Work out the finished part from the listing and answer in its coordinate system (mm). Give positions to 0.01 mm unless a question says otherwise; leave off trailing zeros. Loops run counter-clockwise (first coordinate to the right, second up) from the corner with the lowest first, then second, coordinate; pieces in that order, holes last.
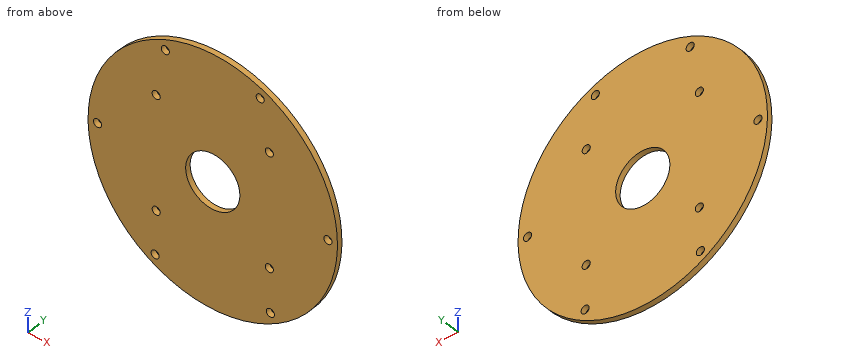
```python
from build123d import *

# Parameters (mm, degrees)
SKETCH_1_R          = 46
EXTRUDE_1_DEPTH     = 2
SKETCH_2_R          = 1.5
CUT_EXTRUDE_1_DEPTH = 66.084560381
SKETCH_3_R          = 1.5
CUT_EXTRUDE_2_DEPTH = 66.084560381
SKETCH_4_R          = 10
CUT_EXTRUDE_3_DEPTH = 66.084560381


with BuildPart() as part:
    # 草图1 → 凸台-拉伸1 (new body)
    with BuildSketch(Plane(origin=(0, 0, 0), x_dir=(1, 0, 0), z_dir=(0, 1, 0))):
        with Locations(Location((0, 0, 0), (0, 0, 270))):
            Circle(SKETCH_1_R)
    extrude(amount=EXTRUDE_1_DEPTH)

    # 草图2 → 切除-拉伸1 (cut, through all)
    with BuildSketch(Plane(origin=(0, 2, 0), x_dir=(1, 0, 0), z_dir=(0, 1, 0))):
        with Locations(Location((-21.25, 36.806079661, 0), (0, 0, 270))):
            Circle(SKETCH_2_R)
        with Locations(Location((21.25, 36.806079661, 0), (0, 0, 270))):
            Circle(SKETCH_2_R)
        with Locations(Location((42.5, 0, 0), (0, 0, 270))):
            Circle(SKETCH_2_R)
        with Locations(Location((-42.5, 0, 0), (0, 0, 270))):
            Circle(SKETCH_2_R)
        with Locations(Location((-17.5, -38.729833462, 0), (0, 0, 270))):
            Circle(SKETCH_2_R)
        with Locations(Location((17.5, -38.729833462, 0), (0, 0, 90))):
            Circle(SKETCH_2_R)
    extrude(amount=-CUT_EXTRUDE_1_DEPTH, mode=Mode.SUBTRACT)

    # 草图3 → 切除-拉伸2 (cut, through all)
    with BuildSketch(Plane(origin=(0, 2, 0), x_dir=(1, 0, 0), z_dir=(0, 1, 0))):
        with Locations(Location((-20.859650045, -20.859650045, 0), (0, 0, 270))):
            Circle(SKETCH_3_R)
        with Locations(Location((-20.859650045, 20.859650045, 0), (0, 0, 270))):
            Circle(SKETCH_3_R)
        with Locations(Location((20.859650045, 20.859650045, 0), (0, 0, 270))):
            Circle(SKETCH_3_R)
        with Locations(Location((20.859650045, -20.859650045, 0), (0, 0, 270))):
            Circle(SKETCH_3_R)
    extrude(amount=-CUT_EXTRUDE_2_DEPTH, mode=Mode.SUBTRACT)

    # 草图4 → 切除-拉伸3 (cut, through all)
    with BuildSketch(Plane(origin=(0, 2, 0), x_dir=(1, 0, 0), z_dir=(0, 1, 0))):
        with Locations(Location((0, 0, 0), (0, 0, 270))):
            Circle(SKETCH_4_R)
    extrude(amount=-CUT_EXTRUDE_3_DEPTH, mode=Mode.SUBTRACT)


solid = part.part
```
Q1. Section D-D on z = -33 is taken. Give the vertices of the cut face in (x, y), plus the area to 3 significant figures.
Q2. Given pin 1 (4 mm diameter, centred on x = -17.5, z = 38.73, fed in from +Y); pin 2 (1 mm diameter, centred on y = 1, z = -19.5, fed in from -X), each flat-ended and moving along its own axis, determine where each tip first touches the part or whether it passes through.
Q3. Consider line 1 along X through (y, z) = (0.2, -38); line 2 along X through (y, z) = (1.25, 38); line 3 along Z through (x, y) = (-19.5, 1.85). Determine where each line is inside the solid, lowest interval first.
Q4. Section C-C on y = 0.65 is taken. State how many separate pieces and enclosed holes the cut face has, plus the area to 3 significant figures.
Q5. Section B-B on z = 7.5 is taken. Give the vertices of the cut face in (x, y).
Q6. Section A-A on x = -17.5 is taken. Give the vertices of the cut face in (y, z).
Check result:
1. outline: (-32.05, 0) - (32.05, 0) - (32.05, 2) - (-32.05, 2) - close
1. area: 128 mm2
2. pin 1: stops at y = 2
2. pin 2: stops at x = -41.89
3. line 1: x = -25.92 to -22.16, -20.34 to 20.34, 22.16 to 25.92
3. line 2: x = -25.92 to -18.81, -16.19 to 16.19, 18.81 to 25.92
3. line 3: z = -41.66 to -21.49, -20.23 to 20.23, 21.49 to 41.66
4. separate pieces: 1
4. enclosed holes: 11
4. area: 6,260 mm2
5. outline: (-45.38, 0) - (-6.61, 0) - (-6.61, 2) - (-45.38, 2) - close; (6.61, 0) - (45.38, 0) - (45.38, 2) - (6.61, 2) - close
6. outline: (0, -42.54) - (2, -42.54) - (2, 37.23) - (0, 37.23) - close; (0, 40.23) - (2, 40.23) - (2, 42.54) - (0, 42.54) - close
